The model under review builds one solid part; all positions refer to its coordinate system, in mm. Face numbers are marked on the shaded views. A direction names the side the tool comes from. Round coordinates to 2 decimals unless told otherwise and drop trailing zeros. Write each loop counter-clockwise with the first axis right and the second up, starting at its lowest first coordinate (ties: lowest second). Pieces come first, ordered by that corner, then holes. Notation, with made-up numbers: (52, 82.5) -> (96, 82.5) arc R17 cw to (96, 110.5) -> close; hole circle Ø5 at (-4, 68). An arc over 180 degrees is marked (long way). Answer as a JSON object with one key per item and string values. Group by question number.
1) We need section A-A, the plane y = 0. Write out the cut boundary in (x, z).
2) We need section D-D, the plane y = -2.25. Write out the cut boundary in (x, z), then the cut area to 3 significant figures.
3) We need section C-C, the plane z = 5.5. Write out the cut boundary in (x, y), then the cut area to 3 significant figures.
4) Insertion check: pin 1 Ø2 at (y, z) = (2.5, 3) entering from -X; pin 2 Ø3 at (y, z) = (1.5, 6.5) entering from +X; pin 3 Ø4 at (y, z) = (-0.5, 21) entering from -X. Each pin has a flat end and moves straight along its axis. Give the tip position at first contact, or say it passes through.
5) Machinability: for the marked faces 1 and 2, which of the approach directions +Z, -Z, +X, -X, +Y, -Y give a long, thin tool a straight path to every point of the face, cutting with its end or side? Answer none if there is none.
6) To check wall thickness, follow probe 1 along Y at (x, z) = (0, 5.5); probe 2 along Z at (x, y) = (2.75, 2); probe 3 along Y at (x, z) = (-1, 21.25). State the ranges of each line that lie inside material, in increasing order. Write a range as [from, to].
7) Mouldability with a two-part tool opening along Y and no side actions: class the marked faces 3, 4 and 5 as pulls with the +Y half, pulls with the -Y half, needs draft (parallel to the pull), parting line crosses it, or undercut.
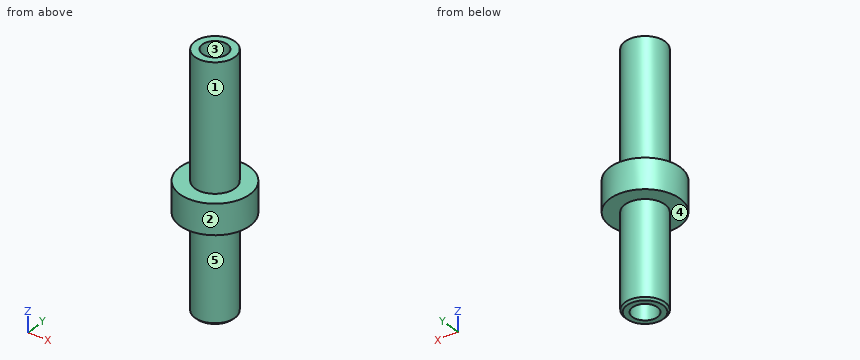
from build123d import *

# Parameters (mm, degrees)
SKETCH_1_R          = 2
EXTRUDE_1_DEPTH     = 25
SKETCH_2_R          = 1.25
CUT_EXTRUDE_1_DEPTH = 26
EXTRUDE_START       = -9.5
SKETCH_3_R          = 3.5
SKETCH_3_R_2        = 2
EXTRUDE_2_DEPTH     = 3
CHAMFER_1_SIZE      = 0.2


with BuildPart() as part:
    # Эскиз1 → Бобышка-Вытянуть1 (new body)
    with BuildSketch(Plane.XY):
        Circle(SKETCH_1_R)
    extrude(amount=EXTRUDE_1_DEPTH)

    # Эскиз2 → Вырез-Вытянуть1 (cut, through all)
    with BuildSketch(Plane.XY.offset(25)):
        Circle(SKETCH_2_R)
    extrude(amount=-CUT_EXTRUDE_1_DEPTH, mode=Mode.SUBTRACT)

    # Эскиз3 → Бобышка-Вытянуть2 (add)
    with BuildSketch(Plane(origin=(0, 0, 0), x_dir=(-1, 0, 0), z_dir=(0, 0, -1)).offset(EXTRUDE_START)):
        Circle(SKETCH_3_R)
        Circle(SKETCH_3_R_2, mode=Mode.SUBTRACT)
    extrude(amount=-EXTRUDE_2_DEPTH)

    # Фаска1
    chamfer_1_edges = [part.edges().sort_by_distance(p)[0] for p in [
        (-2, 0, 0),
    ]]
    chamfer(chamfer_1_edges, length=CHAMFER_1_SIZE)


solid = part.part
Here are the results:
{
 "1": {"outline": "(-3.5, 9.5) -> (-2, 9.5) -> (-2, 0.2) -> (-1.8, 0) -> (-1.25, 0) -> (-1.25, 25) -> (-2, 25) -> (-2, 12.5) -> (-3.5, 12.5) -> close; (1.25, 0) -> (1.8, 0) -> (2, 0.2) -> (2, 9.5) -> (3.5, 9.5) -> (3.5, 12.5) -> (2, 12.5) -> (2, 25) -> (1.25, 25) -> close"},
 "2": {"outline": "(-2.68, 9.5) -> (2.68, 9.5) -> (2.68, 12.5) -> (-2.68, 12.5) -> close", "area": "16.1 mm^2"},
 "3": {"outline": "circle Ø4 at (0, 0); hole circle Ø2.5 at (0, 0)", "area": "7.66 mm^2"},
 "4": {"pin 1": "stops at x = -1.32", "pin 2": "stops at x = 2", "pin 3": "stops at x = -2"},
 "5": {"face 1": "+Z", "face 2": "+Z, -Z"},
 "6": {"probe 1": "y = [-2, -1.25], [1.25, 2]", "probe 2": "z = [9.5, 12.5]", "probe 3": "y = [-1.73, -0.75], [0.75, 1.73]"},
 "7": {"face 3": "undercut", "face 4": "needs draft", "face 5": "parting line crosses it"}
}
